Check sheet for the modelled part. Datum: model origin and axes. Units: mm. Face numbers are marked on the shaded views. A direction names the side the tool comes from. Give positions to 0.01 mm unless a question says otherwise; leave off trailing zeros. Loops run counter-clockwise (first coordinate to the right, second up) from the corner with the lowest first, then second, coordinate; pieces in that order, holes last. Notation, with made-up numbers: (19.5, -36) - (42.5, -36) arc R21 ccw to (42.5, -21) - close; hole circle Ø5 at (50.25, 29.25). An arc over 180 degrees is marked (long way). Answer in a Markdown table with one row per item. Add a question column.
(1) Sectioned sample at C-C on z = 0. State how many separate pieces and enclosed holes the cut face has, then the cut area to 3 significant figures.
(2) Set-up check for the marked faces 1, 2 and 3: record each of +Z, -Z, +X, -X, +Y, -Y from which the full face is reachable in a straight line by a thin tool's end or side.
(3) Go/stop test with flat-tipped pins: P1, Ø3, axis at x = -8.5, z = -0.5, coming from the +Y side; P2, Ø2, axis at x = 3.5, y = -0.5, coming from the +Z side; P3, Ø5.5, axis at x = 0, z = 8, coming from the -Y side; P4, Ø5, axis at x = 0, z = 0, coming from the +Y side. Record where each tip stops, or that it passes through.
(4) Sectioned sample at A-A on y = -1.5. Enter the section's corners in (x, z).
(5) Sectioned sample at D-D on z = 14.75. Enter the section's corners in (x, y).
(6) Thickness scan on L1, parallel to Z at x = 0.5, y = -3.25; L2, parallel to Z at x = 1, y = 2; L3, parallel to X at y = 0.5, z = -1.75. Record the ranges inside material, lowest first.
(7) Sectioned sample at B-B on x = -6.25. Enter the section's corners in (y, z).
from build123d import *

# Parameters (mm, degrees)
BOSS_EXTRUDE1_DEPTH           = 3.9
SKETCH2_R                     = 2.4
CUT_EXTRUDE1_DEPTH            = 25.463442113
SKETCH3_R                     = 3.1
CUT_EXTRUDE2_DEPTH            = 0.8
LPATTERN1_COUNT               = 2
LPATTERN1_PITCH               = 8
LPATTERN1_COPY_1_SKETCH_R     = 3.1
LPATTERN1_COPY_1_DEPTH        = 0.8
LPATTERN1_COL_COUNT           = 2
LPATTERN1_COL_PITCH           = 8
LPATTERN1_COL_COPY_1_SKETCH_R = 3.1
LPATTERN1_COL_COPY_1_DEPTH    = 0.8
LPATTERN2_COUNT               = 3
LPATTERN2_PITCH               = 8
LPATTERN2_COPY_1_SKETCH_R     = 3.1
LPATTERN2_COPY_1_DEPTH        = 0.8
LPATTERN2_COPY_2_SKETCH_R     = 3.1
LPATTERN2_COPY_2_DEPTH        = 0.8
FILLET1_R                     = 2
CHAMFER1_SIZE                 = 0.3


with BuildPart() as part:
    # Sketch1 → Boss-Extrude1 (new, symmetric)
    with BuildSketch(Plane(origin=(0, 0, 0), x_dir=(1, 0, 0), z_dir=(0, 1, 0))):
        with BuildLine():
            Line((-8, -3.9), (8, -3.9))
            ThreePointArc((8, -3.9), (11.9, 0), (8, 3.9))
            Line((8, 3.9), (-8, 3.9))
            ThreePointArc((-8, 3.9), (-11.9, 0), (-8, -3.9))
        make_face()
        with BuildLine():
            Line((-3.9, 0), (-3.9, -16))
            ThreePointArc((-3.9, -16), (0, -19.9), (3.9, -16))
            Line((3.9, -16), (3.9, 0))
            ThreePointArc((3.9, 0), (0, 3.9), (-3.9, 0))
        make_face()
    extrude(amount=BOSS_EXTRUDE1_DEPTH, both=True)

    # Sketch2 → Cut-Extrude1 (cut, through all)
    with BuildSketch(Plane(origin=(0, 3.9, 0), x_dir=(1, 0, 0), z_dir=(0, 1, 0))):
        with Locations(Location((0, 0, 0), (0, 0, 270))):
            Circle(SKETCH2_R)
    cut_extrude1 = extrude(amount=-CUT_EXTRUDE1_DEPTH, mode=Mode.SUBTRACT)

    # Sketch3 → Cut-Extrude2 (cut)
    with BuildSketch(Plane(origin=(0, 3.9, 0), x_dir=(1, 0, 0), z_dir=(0, 1, 0))):
        with Locations(Location((0, 0, 0), (0, 0, 270))):
            Circle(SKETCH3_R)
    cut_extrude2 = extrude(amount=-CUT_EXTRUDE2_DEPTH, mode=Mode.SUBTRACT)

    # Mirror1: Cut-Extrude2 across plane
    add(cut_extrude2.mirror(Plane.ZX), mode=Mode.SUBTRACT)

    # LPattern1: Cut-Extrude1, Cut-Extrude2 ×2
    with Locations(*[(-i * LPATTERN1_PITCH, 0, 0) for i in range(1, LPATTERN1_COUNT)]):
        add(cut_extrude1, mode=Mode.SUBTRACT)
        add(cut_extrude2, mode=Mode.SUBTRACT)

    # LPattern1 copy 1 sketch → LPattern1 copy 1 (cut)
    with BuildSketch(Plane(origin=(-8, -3.9, 0), x_dir=(1, 0, 0), z_dir=(0, -1, 0))):
        Circle(LPATTERN1_COPY_1_SKETCH_R)
    extrude(amount=-LPATTERN1_COPY_1_DEPTH, mode=Mode.SUBTRACT)

    # LPattern1 col: Cut-Extrude1, Cut-Extrude2 ×2
    with Locations(*[(i * LPATTERN1_COL_PITCH, 0, 0) for i in range(1, LPATTERN1_COL_COUNT)]):
        add(cut_extrude1, mode=Mode.SUBTRACT)
        add(cut_extrude2, mode=Mode.SUBTRACT)

    # LPattern1 col copy 1 sketch → LPattern1 col copy 1 (cut)
    with BuildSketch(Plane(origin=(8, -3.9, 0), x_dir=(1, 0, 0), z_dir=(0, -1, 0))):
        Circle(LPATTERN1_COL_COPY_1_SKETCH_R)
    extrude(amount=-LPATTERN1_COL_COPY_1_DEPTH, mode=Mode.SUBTRACT)

    # LPattern2: Cut-Extrude1, Cut-Extrude2 ×3
    with Locations(*[(0, 0, i * LPATTERN2_PITCH) for i in range(1, LPATTERN2_COUNT)]):
        add(cut_extrude1, mode=Mode.SUBTRACT)
        add(cut_extrude2, mode=Mode.SUBTRACT)

    # LPattern2 copy 1 sketch → LPattern2 copy 1 (cut)
    with BuildSketch(Plane(origin=(0, -3.9, 8), x_dir=(1, 0, 0), z_dir=(0, -1, 0))):
        Circle(LPATTERN2_COPY_1_SKETCH_R)
    extrude(amount=-LPATTERN2_COPY_1_DEPTH, mode=Mode.SUBTRACT)

    # LPattern2 copy 2 sketch → LPattern2 copy 2 (cut)
    with BuildSketch(Plane(origin=(0, -3.9, 16), x_dir=(1, 0, 0), z_dir=(0, -1, 0))):
        Circle(LPATTERN2_COPY_2_SKETCH_R)
    extrude(amount=-LPATTERN2_COPY_2_DEPTH, mode=Mode.SUBTRACT)

    # Fillet1
    fillet1_edges = [part.edges().sort_by_distance(p)[0] for p in [
        (3.9, 0, 3.9),
        (-3.9, 0, 3.9),
    ]]
    fillet(fillet1_edges, radius=FILLET1_R)

    # Chamfer1
    chamfer1_edges = [part.edges().sort_by_distance(p)[0] for p in [
        (0, 3.9, 19.9),
        (-3.9, -3.9, 10.95),
        (-3.9, 3.9, 10.95),
        (3.9, -3.9, 10.95),
        (3.9, 3.9, 10.95),
        (6.95, -3.9, 3.9),
        (6.95, 3.9, 3.9),
        (-4.485786438, 3.9, 4.485786438),
        (-4.485786438, -3.9, 4.485786438),
        (4.485786438, 3.9, 4.485786438),
        (4.485786438, -3.9, 4.485786438),
        (-6.95, 3.9, 3.9),
        (11.9, 3.9, 0),
        (0, 3.9, -3.9),
        (-11.9, 3.9, 0),
        (-6.95, -3.9, 3.9),
        (11.9, -3.9, 0),
        (0, -3.9, -3.9),
        (-11.9, -3.9, 0),
        (0, -3.9, 19.9),
    ]]
    chamfer(chamfer1_edges, length=CHAMFER1_SIZE)


solid = part.part
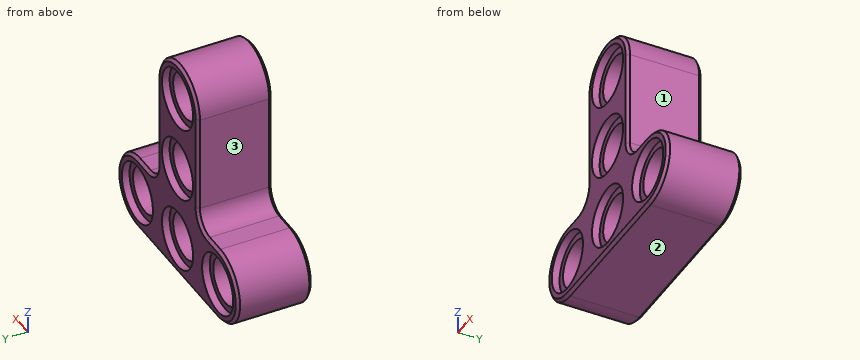
Reply:
| question | item | result |
|---|---|---|
| 1 | separate pieces | 4 |
| 1 | enclosed holes | 0 |
| 1 | area | 66.4 mm^2 |
| 2 | face 1 | +Z, +X, +Y, -Y |
| 2 | face 2 | -Z, +X, -X, +Y, -Y |
| 2 | face 3 | +Z, -X, +Y, -Y |
| 3 | P1 | through |
| 3 | P2 | z = 18.99 |
| 3 | P3 | y = -3.1 |
| 3 | P4 | y = 3.1 |
| 4 | outline | (-8, -3.9) - (8, -3.9) arc R3.9 ccw to (8, 3.9) - (5.9, 3.9) arc R2 cw to (3.9, 5.9) - (3.9, 16) arc R3.9 ccw to (-3.9, 16) - (-3.9, 5.9) arc R2 cw to (-5.9, 3.9) - (-8, 3.9) arc R3.9 ccw to start; hole circle Ø4.8 at (-8, 0); hole circle Ø4.8 at (0, 0); hole circle Ø4.8 at (0, 8); hole circle Ø4.8 at (0, 16); hole circle Ø4.8 at (8, 0) |
| 5 | outline | (-3.9, -3.6) - (-3.6, -3.9) - (-2.84, -3.9) - (-2.84, -3.1) - (-2.05, -3.1) - (-2.05, 3.1) - (-2.84, 3.1) - (-2.84, 3.9) - (-3.6, 3.9) - (-3.9, 3.6) - close; (2.05, -3.1) - (2.84, -3.1) - (2.84, -3.9) - (3.6, -3.9) - (3.9, -3.6) - (3.9, 3.6) - (3.6, 3.9) - (2.84, 3.9) - (2.84, 3.1) - (2.05, 3.1) - close |
| 6 | L1 | -3.9 to -3.06, 3.06 to 4.94, 11.06 to 12.94, 19.06 to 19.87 |
| 6 | L2 | -3.9 to -2.18, 2.18 to 5.82, 10.18 to 13.82, 18.18 to 19.77 |
| 6 | L3 | -11.49 to -9.64, -6.36 to -1.64, 1.64 to 6.36, 9.64 to 11.49 |
| 7 | outline | (-3.9, -3.6) - (-3.6, -3.9) - (3.6, -3.9) - (3.9, -3.6) - (3.9, -2.56) - (3.1, -2.56) - (3.1, -1.64) - (-3.1, -1.64) - (-3.1, -2.56) - (-3.9, -2.56) - close; (-3.9, 2.56) - (-3.1, 2.56) - (-3.1, 1.64) - (3.1, 1.64) - (3.1, 2.56) - (3.9, 2.56) - (3.9, 3.6) - (3.6, 3.9) - (-3.6, 3.9) - (-3.9, 3.6) - close |
